Verification items for the finished model (mm, model axes). A direction names the side the tool comes from. Round coordinates to 2 decimals unless told otherwise and drop trailing zeros. Order: outer loops, then holes, each group sorted by start corner. A loop starts at its lowest first (then second) coordinate and runs counter-clockwise, first axis right, second up. Notation, with made-up numbers: (86, 62.5) -> (101, 62.5) arc R35 ccw to (101, 101.5) -> close; hole circle Ø3 at (71.5, 38.5). An arc over 180 degrees is marked (long way). Put each result on its own line as item: value.
from build123d import *

# Parameters (mm, degrees)
SKETCH1_W           = 34
SKETCH1_H           = 14
BOSS_EXTRUDE1_DEPTH = 2
SKETCH2_W           = 34
SKETCH2_H           = 7
BOSS_EXTRUDE2_DEPTH = 5
FILLET1_R           = 0.5
CUT_EXTRUDE1_REACH  = 21.053
SKETCH3_R           = 1.25


with BuildPart() as part:
    # Sketch1 → Boss-Extrude1 (new body)
    with BuildSketch(Plane(origin=(0, 0, 0), x_dir=(1, 0, 0), z_dir=(0, 1, 0))):
        Rectangle(SKETCH1_W, SKETCH1_H)
    extrude(amount=BOSS_EXTRUDE1_DEPTH)

    # Sketch2 → Boss-Extrude2 (add)
    with BuildSketch(Plane(origin=(0, 2, 0), x_dir=(1, 0, 0), z_dir=(0, 1, 0))):
        with Locations((0, -3.5)):
            Rectangle(SKETCH2_W, SKETCH2_H)
    extrude(amount=BOSS_EXTRUDE2_DEPTH)

    # Fillet1
    fillet1_edges = [part.edges().sort_by_distance(p)[0] for p in [
        (17, 4.5, 0),
        (-17, 4.5, 0),
        (17, 3.5, 7),
        (-17, 3.5, 7),
        (-17, 1, -7),
        (17, 1, -7),
    ]]
    fillet(fillet1_edges, radius=FILLET1_R)

    # Sketch3 → Cut-Extrude1 (cut, up to next)
    with BuildSketch(Plane(origin=(0, 2, 0), x_dir=(1, 0, 0), z_dir=(0, 1, 0)), mode=Mode.PRIVATE) as cut_extrude1_sk1:
        with Locations(Location((12, 3.5, 0), (0, 0, 270))):
            Circle(SKETCH3_R)
    cut_extrude1_tool1 = extrude(cut_extrude1_sk1.sketch, amount=-CUT_EXTRUDE1_REACH, mode=Mode.PRIVATE) & part.part
    # Sketch3 → Cut-Extrude1 (cut, up to next)
    with BuildSketch(Plane(origin=(0, 2, 0), x_dir=(1, 0, 0), z_dir=(0, 1, 0)), mode=Mode.PRIVATE) as cut_extrude1_sk2:
        with Locations(Location((-12, 3.5, 0), (0, 0, 270))):
            Circle(SKETCH3_R)
    cut_extrude1_tool2 = extrude(cut_extrude1_sk2.sketch, amount=-CUT_EXTRUDE1_REACH, mode=Mode.PRIVATE) & part.part
    add(cut_extrude1_tool1.solids().sort_by_distance((12, 2, -3.5))[0], mode=Mode.SUBTRACT)
    add(cut_extrude1_tool2.solids().sort_by_distance((-12, 2, -3.5))[0], mode=Mode.SUBTRACT)


solid = part.part
Item 1: Material ranges on L1, parallel to X at y = 0.8, z = -3.5; L2, parallel to X at y = 0.5, z = -3; L3, parallel to Y at x = 14.5, z = -4.5, recorded low to high. Write a range as [from, to].
Check sheet entries:
L1: x = [-17, -13.25], [-10.75, 10.75], [13.25, 17]
L2: x = [-17, -13.15], [-10.85, 10.85], [13.15, 17]
L3: y = [0, 2]
Item 2: Section check B-B on z = -3.5. Record the boundary of the cut face in (x, y), then the cut area to 3 significant figures.
Check sheet entries:
outline: (-17, 0) -> (-13.25, 0) -> (-13.25, 2) -> (-17, 2) -> close; (-10.75, 0) -> (10.75, 0) -> (10.75, 2) -> (-10.75, 2) -> close; (13.25, 0) -> (17, 0) -> (17, 2) -> (13.25, 2) -> close
area: 58.0 mm^2
Item 3: Gauge pin test, flat ends, axial feed: pin 1 Ø4 at (x, y) = (-4.5, 6) entering from -Z; pin 2 Ø1.5 at (x, z) = (12, -3.5) entering from +Y; pin 3 Ø4 at (x, z) = (-12, -3.5) entering from +Y. Record the tip position at first contact, or that the pin passes through.
Check sheet entries:
pin 1: stops at z = 0
pin 2: passes through
pin 3: stops at y = 2
Item 4: Release check for a two-part mould opening along X. For faces 3 (the flat face through (0, 0, 0)), 4 (the flat face through (17, 3, 2)), 5 (the cylindrical face through (13.054, 1.014, -2.828)) record: +X half, -X half, draft (parallel to the pull), parting line (faces both ways), or undercut.
Check sheet entries:
face 3: draft
face 4: +X half
face 5: undercut
Item 5: Section check C-C on y = 5.5. Record the boundary of the cut face in (x, z).
Check sheet entries:
outline: (-17, 0.5) arc R0.5 ccw to (-16.5, 0) -> (16.5, 0) arc R0.5 ccw to (17, 0.5) -> (17, 6.5) arc R0.5 ccw to (16.5, 7) -> (-16.5, 7) arc R0.5 ccw to (-17, 6.5) -> close
Item 6: Section check D-D on x = 10. Record the boundary of the cut face in (y, z).
Check sheet entries:
outline: (0, -7) -> (2, -7) -> (2, 0) -> (7, 0) -> (7, 7) -> (0, 7) -> close
Item 7: Section check A-A on x = -12. Record the boundary of the cut face in (y, z), then the cut area to 3 significant figures.
Check sheet entries:
outline: (0, -7) -> (2, -7) -> (2, -4.75) -> (0, -4.75) -> close; (0, -2.25) -> (2, -2.25) -> (2, 0) -> (7, 0) -> (7, 7) -> (0, 7) -> close
area: 58.0 mm^2
Item 8: Tool access check on faces 1 (the flat face through (-17, 3, 2)), 2 (the flat face through (0, 4, 0)). Record the directions out of +Z, -Z, +X, -X, +Y, -Y that give a thin tool (end or side, any length) a straight path to the whole face; none if there is none.
Check sheet entries:
face 1: +Z, -Z, -X, +Y, -Y
face 2: -Z, +X, -X, +Y
